Autodesk Inventor part; units mm, degrees
ref_plane "YZ Plane" through (0, 0, 0) normal (1, 0, 0) x (0, 1, 0)
ref_plane "XZ Plane" through (0, 0, 0) normal (0, 1, 0) x (-1, 0, 0)
ref_plane "XY Plane" through (0, 0, 0) normal (0, 0, 1) x (1, 0, 0)
sketch "Sketch1" plane through (0, 0, 0) normal (0, 1, 0) x (-1, 0, 0)
  line L0 (35, 27.5) -> (-35, 27.5)
  line L1 (-35, 27.5) -> (-35, -27.5)
  line L2 (-35, -27.5) -> (35, -27.5)
  line L3 (35, -27.5) -> (35, 27.5)
  line L4 (35, 27.5) -> (-35, -27.5) construction
  line L5 (-35, 27.5) -> (35, -27.5) construction
  point P0 (0, 0)
  dimension "d0" = 70
  dimension "d1" = 55
extrude "Extrusion1" add sketch "Sketch1" along normal blind 5
sketch "Sketch2" plane through (0, 5, 0) normal (0, 1, 0) x (1, 0, 0)
  circle A0 centre (-30, 22.5) radius 2.1
  circle A1 centre (30, 22.5) radius 2.1
  line L0 (35, 27.5) -> (-35, 27.5)
  line L1 (-35, 27.5) -> (-35, -27.5)
  line L2 (35, -27.5) -> (35, 27.5)
  point P0 (0, 0)
  dimension "d4" = 4.2
  dimension "d5" = 4.2
  dimension "d6" = 5
  dimension "d7" = 5
  dimension "d8" = 5
  dimension "d9" = 5
extrude "Extrusion2" cut sketch "Sketch2" against normal blind 5
sketch "Sketch3" plane through (0, 5, 0) normal (0, 1, 0) x (1, 0, 0)
  line L0 (-35, -27.5) -> (35, -27.5)
  line L1 (35, -27.5) -> (35, -21.3758)
  line L2 (35, -21.3758) -> (-35, -21.3758)
  line L3 (-35, -21.3758) -> (-35, -27.5)
  line L4 (-35, -27.5) -> (35, -21.3758) construction
  line L5 (35, -27.5) -> (-35, -21.3758) construction
  line L6 (-35, -27.5) -> (35, -27.5)
  line L7 (35, -27.5) -> (35, 27.5)
  line L8 (-35, 27.5) -> (-35, -27.5)
  point P0 (0, 0)
  point P1 (0, -24.4379)
  dimension "d12" = 5
extrude "Extrusion3" add sketch "Sketch3" along normal blind 60
sketch "Sketch4" plane through (-35, 0, 27.5) normal (0, 0, 1) x (1, 0, 0)
  circle A0 centre (21, 49) radius 1.05
  circle A1 centre (49, 49) radius 1.05
  circle A2 centre (21, 21) radius 1.05
  circle A3 centre (49, 21) radius 1.05
  line L0 (0, 0) -> (70, 0)
  line L1 (70, 0) -> (70, 65)
  line L2 (0, 0) -> (0, 65)
  point P0 (35, 0)
  dimension "d15" = 2.1
  dimension "d16" = 2.1
  dimension "d17" = 2.1
  dimension "d18" = 2.1
  dimension "d19" = 21
  dimension "d20" = 21
  dimension "d21" = 21
  dimension "d22" = 28
extrude "Extrusion4" cut sketch "Sketch4" against normal blind 50
sketch "Sketch5" plane through (-35, 0, 27.5) normal (0, 0, 1) x (1, 0, 0)
  line L0 (27.5, 16) -> (42.5, 16)
  line L1 (42.5, 16) -> (42.5, 26)
  line L2 (42.5, 26) -> (27.5, 26)
  line L3 (27.5, 26) -> (27.5, 16)
  line L4 (27.5, 16) -> (42.5, 26) construction
  line L5 (42.5, 16) -> (27.5, 26) construction
  line L6 (0, 0) -> (70, 0)
  point P0 (35, 0)
  point P1 (35, 21)
  point P2 (35, 0)
  dimension "d25" = 15
  dimension "d26" = 10
  dimension "d27" = 21
extrude "Extrusion5" cut sketch "Sketch5" against normal blind 50
properties part number "camera_bottom"
Verification items for the finished model (mm, model axes). A direction names the side the tool comes from. Coordinates: 2 decimals unless noted, no trailing zeros. Write each loop counter-clockwise with the first axis right and the second up, starting at its lowest first coordinate (ties: lowest second). Pieces come first, ordered by that corner, then holes. Notation, with made-up numbers: M 18.5,35 L 64.5,35 A11 ccw 64.5,43 Z; hole C -10.5,22.5 d2. An arc over 180 degrees is marked long. Use CSV: the item, a comma, the result in double quotes.
Q1. Go/stop test with flat-tipped pins: P1, Ø2, axis at x = -11.5, y = 55.5, coming from the -Z side; P2, Ø14.5, axis at x = -4.5, z = 4, coming from the +Y side. Record where each tip stops, or that it passes through.
Computed values:
P1,"z = 21.38"
P2,"y = 5"
Q2. Section check C-C, the plane y = 49. Enter the section's corners in (x, z).
Computed values:
outline,"M -35,21.38 L -15.05,21.38 L -15.05,27.5 L -35,27.5 Z; M -12.95,21.38 L 12.95,21.38 L 12.95,27.5 L -12.95,27.5 Z; M 15.05,21.38 L 35,21.38 L 35,27.5 L 15.05,27.5 Z"
Q3. Set-up check for faces 1 (the flat face through (0, 35, 21.376)), 2 (the flat face through (0, 26, 24)), 3 (the cylindrical face through (27.9, 2.54, -22.59)): record each of +Z, -Z, +X, -X, +Y, -Y from which the full face is reachable in a straight line by a thin tool's end or side.
Computed values:
face 1,"-Z, +X, -X, +Y"
face 2,"+Z, -Z"
face 3,"+Y, -Y"
Q4. Section check A-A, the plane x = -14. Enter the section's corners in (y, z).
Computed values:
outline,"M 0,-27.5 L 5,-27.5 L 5,21.38 L 19.95,21.38 L 19.95,27.5 L 0,27.5 Z; M 22.05,21.38 L 47.95,21.38 L 47.95,27.5 L 22.05,27.5 Z; M 50.05,21.38 L 65,21.38 L 65,27.5 L 50.05,27.5 Z"
Q5. Thickness scan on line 1 along Y through (x, z) = (14, 23.25); line 2 along Z through (x, y) = (30, 1); line 3 along Z through (x, y) = (-20, 54). Record the ranges inside material, lowest first. Write a range as [from, to].
Computed values:
line 1,"[0, 19.95], [22.05, 47.95], [50.05, 65]"
line 2,"[-27.5, -24.6], [-20.4, 27.5]"
line 3,"[21.38, 27.5]"
Q6. Section check B-B, the plane z = -22.5. Enter the section's corners in (x, y).
Computed values:
outline,"M -35,0 L -32.1,0 L -32.1,5 L -35,5 Z; M -27.9,0 L 27.9,0 L 27.9,5 L -27.9,5 Z; M 32.1,0 L 35,0 L 35,5 L 32.1,5 Z"
Q7. Section check D-D, the plane x = -30. Enter the section's corners in (y, z), and give its area (3 significant figures).
Computed values:
outline,"M 0,-27.5 L 5,-27.5 L 5,-24.6 L 0,-24.6 Z; M 0,-20.4 L 5,-20.4 L 5,21.38 L 65,21.38 L 65,27.5 L 0,27.5 Z"
area,"621 mm²"
Q8. Mould release check, pull along X, two halves, no side actions. Record for faces 4 (the flat face through (-35, 20, 22)), 5 (the flat face through (0, 2, -27.5)), 6 (the flat face through (7.5, 21, 24)): pulls with the +X half, pulls with the -X half, needs draft (parallel to the pull), parting line crosses it, or undercut.
Computed values:
face 4,"pulls with the -X half"
face 5,"needs draft"
face 6,"undercut"
